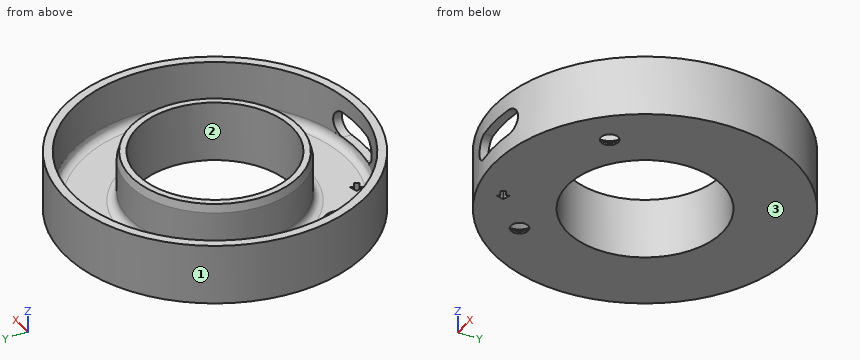
```python
from build123d import *

# Parameters (mm, degrees)
CROQUIS1_R              = 35
SALIENTE_EXTRUIR1_DEPTH = 14
CROQUIS2_R              = 18
CORTAR_EXTRUIR1_DEPTH   = 52.439284598
VACIADO1_T              = -2
REDONDEO1_R             = 2
CORTAR_EXTRUIR2_START   = -22
CORTAR_EXTRUIR2_DEPTH   = 30.439284598
CROQUIS4_R              = 2
CORTAR_EXTRUIR3_DEPTH   = 51.931326474
CHAFL_N1_SIZE           = 1.5
CHAFL_N2_SIZE           = 0.5
CHAFL_N2_SIZE2          = 1.866025404


with BuildPart() as part:
    # Croquis1 → Saliente-Extruir1 (new body)
    with BuildSketch(Plane.XY):
        Circle(CROQUIS1_R)
    extrude(amount=SALIENTE_EXTRUIR1_DEPTH)

    # Croquis2 → Cortar-Extruir1 (cut, through all)
    with BuildSketch(Plane.XY.offset(14)):
        Circle(CROQUIS2_R)
    extrude(amount=-CORTAR_EXTRUIR1_DEPTH, mode=Mode.SUBTRACT)

    # Vaciado1
    vaciado1_openings = [part.faces().sort_by_distance(p)[0] for p in [
        (-34.010050506, 0, 14),
    ]]
    offset(amount=VACIADO1_T, openings=vaciado1_openings, kind=Kind.INTERSECTION)

    # Redondeo1
    redondeo1_edges = [part.edges().sort_by_distance(p)[0] for p in [
        (-33, 0, 2),
        (-20, 0, 2),
    ]]
    fillet(redondeo1_edges, radius=REDONDEO1_R)

    # Croquis3 → Cortar-Extruir2 (cut, through all)
    with BuildSketch(Plane(origin=(0, 0, 0), x_dir=(1, 0, 0), z_dir=(0, 1, 0)).offset(CORTAR_EXTRUIR2_START)):
        with BuildLine():
            Line((-5, -4), (5, -4))
            ThreePointArc((5, -4), (8, -7), (5, -10))
            Line((5, -10), (-5, -10))
            ThreePointArc((-5, -10), (-8, -7), (-5, -4))
        make_face()
    extrude(amount=-CORTAR_EXTRUIR2_DEPTH, mode=Mode.SUBTRACT)

    # Croquis4 → Cortar-Extruir3 (cut, through all)
    with BuildSketch(Plane.XY.offset(2)):
        with Locations((-18.738329701, -18.738329701)):
            Circle(CROQUIS4_R)
        with Locations((18.738329701, -18.738329701)):
            Circle(CROQUIS4_R)
        Polygon((-8.115597392, -27.870752521), (-9.499112417, -27.112050733), (-9.05906538, -26.309612019), (-10.984489851, -26.871194156), (-10.422907714, -28.796618627), (-10.021777616, -28.065146095), (-8.638262591, -28.823847883), align=None)
    extrude(amount=-CORTAR_EXTRUIR3_DEPTH, mode=Mode.SUBTRACT)

    # Chaflán1
    chafl_n1_edges = [part.edges().sort_by_distance(p)[0] for p in [
        (-20.738329701, -18.738329701, 2),
        (16.738329701, -18.738329701, 2),
    ]]
    chamfer(chafl_n1_edges, length=CHAFL_N1_SIZE)

    # Chaflán2
    chafl_n2_edges = [part.edges().sort_by_distance(p)[0] for p in [
        (-20, 0, 14),
    ]]
    chafl_n2_side = [part.faces().sort_by_distance(p)[0] for p in [
        (-19.434314575, 0, 14),
    ]]
    chamfer(chafl_n2_edges, length=CHAFL_N2_SIZE, length2=CHAFL_N2_SIZE2, reference=chafl_n2_side[0])


solid = part.part
```
Can you work these out from the model? Positions are in its coordinate system, mm. Face numbers are marked on the shaded views. Round coordinates to 2 decimals unless told otherwise and drop trailing zeros. Loops run counter-clockwise (first coordinate to the right, second up) from the corner with the lowest first, then second, coordinate; pieces in that order, holes last. Notation, with made-up numbers: M 58,31 L 67,31 A27 cw 67,59 Z; hole C 64.5,30.5 d6. An arc over 180 degrees is marked long. Answer as a JSON object with one key per item and string values. Group by question number.
Q1. We'd pull the mould along Y, two halves only. Please class the marked faces 1, 2 and 3: +Y half, -Y half, draft (parallel to the pull), parting line (faces both ways), or undercut.
Q2. Will these pins go through, and if not, where does the flat tip stop? pin 1 (1.5 mm diameter, centred on x = -2.5, z = 4.5, fed in from +Y); pin 2 (4 mm diameter, centred on y = -19, z = 2.5, fed in from +X); pin 3 (5 mm diameter, centred on y = -21, z = 7, fed in from +X).
Q3. Imagine slicing it at C-C, the plane z = 8. Please give me the cut outline in (x, y), then the cut area to 3 significant figures.
Q4. Imagine slicing it at D-D, the plane z = 3. Please give me the cut outline in (x, y), then the cut area to 3 significant figures.
Q5. Imagine slicing it at B-B, the plane y = 0. Please give me the cut outline in (x, z).
Q6. Imagine slicing it at A-A, the plane x = 0. Please give me the cut outline in (y, z), then the cut area to 3 significant figures.
Q7. Please list where these lines run through material, in increasing order: L1, parallel to Y at x = 0, z = 9.5; L2, parallel to Y at x = 12.5, z = 11.5; L3, parallel to Y at x = -2, z = 9.75.
Findings:
{
 "1": {"face 1": "parting line", "face 2": "undercut", "face 3": "draft"},
 "2": {"pin 1": "stops at y = 34.96", "pin 2": "stops at x = 30.59", "pin 3": "stops at x = 29.71"},
 "3": {"outline": "C 0,0 d40; M -7.83,-34.11 L -7.83,-32.06 A33 cw long 7.83,-32.06 L 7.83,-34.11 A35 ccw long Z; hole C 0,0 d36", "area": "634 mm2"},
 "4": {"outline": "C 0,0 d70; C 0,0 d40.54; hole C 0,0 d65.46; hole C 0,0 d36", "area": "755 mm2"},
 "5": {"outline": "M -35,0 L -18,0 L -18,14 L -19.5,14 L -20,12.13 L -20,4 A2 cw -22,2 L -31,2 A2 cw -33,4 L -33,14 L -35,14 Z; M 18,0 L 35,0 L 35,14 L 33,14 L 33,4 A2 cw 31,2 L 22,2 A2 cw 20,4 L 20,12.13 L 19.5,14 L 18,14 Z"},
 "6": {"outline": "M -35,0 L -18,0 L -18,14 L -19.5,14 L -20,12.13 L -20,4 A2 cw -22,2 L -31,2 A2 cw -33,4 L -35,4 Z; M -35,10 L -33,10 L -33,14 L -35,14 Z; M 18,0 L 35,0 L 35,14 L 33,14 L 33,4 A2 cw 31,2 L 22,2 A2 cw 20,4 L 20,12.13 L 19.5,14 L 18,14 Z", "area": "155 mm2"},
 "7": {"L1": "y = -20 to -18, 18 to 20, 33 to 35", "L2": "y = -32.69 to -30.54, -15.61 to -12.95, 12.95 to 15.61, 30.54 to 32.69", "L3": "y = -19.9 to -17.89, 17.89 to 19.9, 32.94 to 34.94"}
}
